```python
from build123d import *

# Parameters (mm, degrees)
SKETCH_1_R               = 50
EXTRUDE_1_DEPTH          = 3
PATTERN_CIRCULAR_1_COUNT = 6
SKETCH_7_R               = 15
CUT_EXTRUDE_1_DEPTH      = 3
CHAMFER_1_SIZE           = 1


with BuildPart() as part:
    # 草图1 → 凸台-拉伸1 (new body)
    with BuildSketch(Plane(origin=(0, 0, 0), x_dir=(1, 0, 0), z_dir=(0, 1, 0))):
        with Locations(Location((0, 0, 0), (0, 0, 270))):
            Circle(SKETCH_1_R)
    extrude(amount=EXTRUDE_1_DEPTH)

    # 草图6 → M8 螺纹孔的螺纹孔钻头1 (revolve, cut)
    with BuildSketch(Plane(origin=(0, 0, 40), x_dir=(0, 0, -1), z_dir=(1, 0, 0))):
        Polygon((0, 0), (0, 18.042926105), (3.4, 16), (3.4, 0), align=None)
    hole_wizard_m8_1 = revolve(axis=Axis((0, -6.35, 40), (0, 1, 0)), mode=Mode.SUBTRACT)

    # 阵列(圆周)1: M8 螺纹孔的螺纹孔钻头1 ×6 about axis
    pattern_circular_1_axis = Axis((0, 0, 0), (0, 1, 0))
    for i in range(1, PATTERN_CIRCULAR_1_COUNT):
        add(hole_wizard_m8_1.rotate(pattern_circular_1_axis, i * 360 / PATTERN_CIRCULAR_1_COUNT), mode=Mode.SUBTRACT)

    # 草图7 → 切除-拉伸1 (cut)
    with BuildSketch(Plane.XZ):
        with Locations(Location((0, 0, 0), (0, 0, 270))):
            Circle(SKETCH_7_R)
    extrude(amount=-CUT_EXTRUDE_1_DEPTH, mode=Mode.SUBTRACT)

    # 倒角1
    chamfer_1_edges = [part.edges().sort_by_distance(p)[0] for p in [
        (0, 0, -50),
        (0, 3, 15),
        (0, 0, 15),
        (0, 3, -50),
    ]]
    chamfer(chamfer_1_edges, length=CHAMFER_1_SIZE)


solid = part.part
```
Work out the finished part from the listing and answer in its coordinate system (mm). Round coordinates to 2 decimals unless told otherwise and drop trailing zeros. Write each loop counter-clockwise with the first axis right and the second up, starting at its lowest first coordinate (ties: lowest second). Pieces come first, ordered by that corner, then holes.
1) A cutting plane is placed at C-C on z = -20. Give the number of separate pieces and of enclosed holes in the cut face, and give its area (3 significant figures).
2) A cutting plane is placed at B-B on z = 0. Determine the outline of the cut face in (x, y).
3) A cutting plane is placed at A-A on x = 0. Determine the outline of the cut face in (y, z).
4) Determine the mould class of faces 1 (the face through (15.02, 1.49, 47.69)), 2 (the face through (12, 0, -12)), 3 (the face through (-38.012, 1.479, -19.557)) for opening direction X: pulls with the +X half, pulls with the -X half, needs draft (parallel to the pull), parting line crosses it, or undercut.
5) A flat-ended cylindrical pin translates along its axis: P1, Ø4, axis at x = -34.64, z = -20, coming from the +Y side. Find the tip coordinate at first contact, or state that the pin passes through.
6) Consider probe 1 along X at (y, z) = (1.25, -20); probe 2 along X at (y, z) = (0.2, -17.5); probe 3 along Z at (x, y) = (34.5, 1.05). Determine where each line is inside the solid, lowest interval first.
Entries:
1. separate pieces: 3
1. enclosed holes: 0
1. area: 232 mm2
2. outline: (-50, 1) - (-49, 0) - (-16, 0) - (-15, 1) - (-15, 2) - (-16, 3) - (-49, 3) - (-50, 2) - close; (15, 1) - (16, 0) - (49, 0) - (50, 1) - (50, 2) - (49, 3) - (16, 3) - (15, 2) - close
3. outline: (0, -49) - (1, -50) - (2, -50) - (3, -49) - (3, -43.4) - (0, -43.4) - close; (0, -36.6) - (3, -36.6) - (3, -16) - (2, -15) - (1, -15) - (0, -16) - close; (0, 16) - (1, 15) - (2, 15) - (3, 16) - (3, 36.6) - (0, 36.6) - close; (0, 43.4) - (3, 43.4) - (3, 49) - (2, 50) - (1, 50) - (0, 49) - close
4. face 1: parting line crosses it
4. face 2: needs draft
4. face 3: undercut
5. P1: passes through
6. probe 1: x = -45.83 to -38.04, -31.24 to 31.24, 38.04 to 45.83
6. probe 2: x = -45.98 to -36.95, -32.34 to 32.34, 36.95 to 45.98
6. probe 3: z = -36.19 to -23.4, -16.6 to 16.6, 23.4 to 36.19
